Build history of the part. All positions in model axes, mm. Face numbers are marked on the shaded views. A direction names the side the tool comes from. Round coordinates to 2 decimals unless told otherwise and drop trailing zeros. Loops run counter-clockwise (first coordinate to the right, second up) from the corner with the lowest first, then second, coordinate; pieces in that order, holes last. Notation, with made-up numbers: (-4, -33.5) -> (43, -33.5) arc R30 ccw to (43, -1.5) -> close; hole circle Ø8 at (-27.75, 82). An arc over 180 degrees is marked (long way). Put each result on its own line as item: value. Start each with the question number.
Item 1: Cut at C-C, the plane y = 11.59. List the corners of the cut face in (x, z) (3 decimals).
Item 2: Tool access for the marked faces 1, 2 and 3: list every direction of +Z, -Z, +X, -X, +Y, -Y with a clear straight run to the whole face (end or side of a thin tool).
Item 3: Pull direction Y, two halves, no side cores. Call the marked faces 4, 5 and 6: +Y half, -Y half, draft (parallel to the pull), parting line (faces both ways), or undercut.
Item 4: Cut at B-B, the plane x = 3. List the corners of the cut face in (y, z), plus the area to 3 significant figures.
Item 5: Cut at D-D, the plane x = 20. List the corners of the cut face in (y, z).
Item 6: Drill centre lines: probe 1 along Y at (x, z) = (-26, 2); probe 2 along Y at (x, z) = (-4, 6.5); probe 3 along X at (y, z) = (2, 9.25). Where is each one in solid material? Low to high. Write a range as [from, to].
Item 7: Flat gauge pins, fed straight in: pin 1 Ø3 at (x, z) = (21.5, 3.5) entering from -Y; pin 2 Ø2.5 at (x, z) = (23, 8) entering from -Y; pin 3 Ø4 at (x, z) = (-24, 4.5) entering from +Y. Where does each tip first touch, or does it go through?
Item 8: Cut at A-A, the plane y = 38.79. List the corners of the cut face in (x, z) (3 decimals).
```python
from build123d import *

# Parameters (mm, degrees)
SKETCH007_W                               = 14.824166
SKETCH007_H                               = 2.145144
EXTRUDE007_DEPTH                          = 7
SKETCH006_W                               = 3.554402
SKETCH006_H                               = 1.424327
EXTRUDE006_DEPTH                          = 10
SKETCH004_AS_DRAWN_W                      = 3.541569
SKETCH004_AS_DRAWN_H                      = 1.411495
EXTRUDE005_DEPTH                          = 7
EXTRUDE005_ONTO_SKETCH004_ROLL_ANGLE      = 90
EXTRUDE005_ONTO_SKETCH004_PLACEMENT_ANGLE = 147.47511
SKETCH005_W                               = 3.573389
SKETCH005_H                               = 1.465404
EXTRUDE004_DEPTH                          = 10
SKETCH003_AS_DRAWN_W                      = 3.579881
SKETCH003_AS_DRAWN_H                      = 1.40319
EXTRUDE003_DEPTH                          = 7
EXTRUDE003_ONTO_SKETCH003_ROLL_ANGLE      = 90
EXTRUDE003_ONTO_SKETCH003_PLACEMENT_ANGLE = -147.47511
EXTRUDE002_DEPTH                          = 5
SKETCH_R                                  = 1.75
EXTRUDE_DEPTH                             = 12


with BuildPart() as extrude007:
    # Sketch007 (on Face32 of Cut004) → Extrude007 (new body)
    with BuildSketch(Plane(origin=(24, 0, 0), x_dir=(0, -1, 0), z_dir=(-1, 0, 0))):
        with Locations((-23.062542, 8.033458)):
            Rectangle(SKETCH007_W, SKETCH007_H)
    extrude(amount=-EXTRUDE007_DEPTH)


with BuildPart() as extrude006:
    # Sketch006 (on Face23 of Cut002) → Extrude006 (new body)
    with BuildSketch(Plane.XZ.offset(-36.8)):
        with Locations((-19.910848, 8.431245)):
            Rectangle(SKETCH006_W, SKETCH006_H)
    extrude(amount=-EXTRUDE006_DEPTH)


with BuildPart() as extrude005:
    # Sketch004 as drawn → Extrude005 (new)
    with BuildSketch(Plane.XY):
        with Locations((9.550918, 8.438737)):
            Rectangle(SKETCH004_AS_DRAWN_W, SKETCH004_AS_DRAWN_H)
    extrude(amount=-EXTRUDE005_DEPTH)


with BuildPart() as extrude005_1:
    # Extrude005 onto Sketch004 roll: moved
    add(extrude005.part.rotate(Axis((0, 0, 0), (1, 0, 0)), EXTRUDE005_ONTO_SKETCH004_ROLL_ANGLE))


with BuildPart() as extrude005_2:
    # Extrude005 onto Sketch004 placement: moved
    add(extrude005_1.part.moved(Location((-2.303479, -3.612274, 0))).rotate(Axis((-2.303479, -3.612274, 0), (0, 0, 1)), EXTRUDE005_ONTO_SKETCH004_PLACEMENT_ANGLE))


with BuildPart() as extrude004:
    # Sketch005 (on Face23 of Cut001) → Extrude004 (new body)
    with BuildSketch(Plane.XZ.offset(-36.8)):
        with Locations((19.895352, 8.368902)):
            Rectangle(SKETCH005_W, SKETCH005_H)
    extrude(amount=-EXTRUDE004_DEPTH)


with BuildPart() as extrude003:
    # Sketch003 as drawn → Extrude003 (new)
    with BuildSketch(Plane.XY):
        with Locations((-9.548731, 8.412013)):
            Rectangle(SKETCH003_AS_DRAWN_W, SKETCH003_AS_DRAWN_H)
    extrude(amount=-EXTRUDE003_DEPTH)


with BuildPart() as extrude003_1:
    # Extrude003 onto Sketch003 roll: moved
    add(extrude003.part.rotate(Axis((0, 0, 0), (1, 0, 0)), EXTRUDE003_ONTO_SKETCH003_ROLL_ANGLE))


with BuildPart() as extrude003_2:
    # Extrude003 onto Sketch003 placement: moved
    add(extrude003_1.part.moved(Location((2.303479, -3.612274, 0))).rotate(Axis((2.303479, -3.612274, 0), (0, 0, 1)), EXTRUDE003_ONTO_SKETCH003_PLACEMENT_ANGLE))


with BuildPart() as extrude002:
    # Sketch002 (on Face4 of Extrude) → Extrude002 (new body)
    with BuildSketch(Plane.YZ.offset(29)):
        with BuildLine():
            ThreePointArc((13.665, 7.65), (11.59, 9.725), (9.515, 7.65))
            Line((9.515, 7.65), (9.515, 2.15))
            ThreePointArc((9.515, 2.15), (11.59, 0.075), (13.665, 2.15))
            Line((13.665, 2.15), (13.665, 7.65))
        make_face()
    extrude(amount=-EXTRUDE002_DEPTH)


with BuildPart() as cut005:
    # Sketch → Extrude (new body)
    with BuildSketch(Plane.XY):
        Polygon((-21, 46.4), (21, 46.4), (21, 41.8), (29, 41.8), (29, -0.2), (21, -0.2), (6.4, -6), (-6.4, -6), (-21, -0.2), (-29, -0.2), (-29, 41.8), (-21, 41.8), align=None)
        with Locations((-25.875, 38.79)):
            Circle(SKETCH_R, mode=Mode.SUBTRACT)
        with Locations((25.875, 38.79)):
            Circle(SKETCH_R, mode=Mode.SUBTRACT)
        with Locations((25.875, 2.81)):
            Circle(SKETCH_R, mode=Mode.SUBTRACT)
        with Locations((-25.875, 2.81)):
            Circle(SKETCH_R, mode=Mode.SUBTRACT)
        with BuildLine():
            Line((-16, 41.4), (16, 41.4))
            Line((16, 41.4), (16, 36.8))
            Line((16, 36.8), (24, 36.8))
            Line((24, 36.8), (24, 4.8))
            Line((24, 4.8), (16, 4.8))
            ThreePointArc((16, 4.8), (14.479309, 4.429189), (13.3, 3.4))
            Line((6.4, -1), (13.3, 3.4))
            Line((-6.4, -1), (6.4, -1))
            Line((-6.4, -1), (-13.3, 3.4))
            ThreePointArc((-13.3, 3.4), (-14.479309, 4.429189), (-16, 4.8))
            Line((-24, 4.8), (-16, 4.8))
            Line((-24, 36.8), (-24, 4.8))
            Line((-16, 36.8), (-24, 36.8))
            Line((-16, 41.4), (-16, 36.8))
        make_face(mode=Mode.SUBTRACT)
    extrude(amount=EXTRUDE_DEPTH)

    # Cut: cut Extrude002
    add(extrude002.part, mode=Mode.SUBTRACT)

    # Cut001: cut Extrude003
    add(extrude003_2.part, mode=Mode.SUBTRACT)

    # Cut002: cut Extrude004
    add(extrude004.part, mode=Mode.SUBTRACT)

    # Cut003: cut Extrude005
    add(extrude005_2.part, mode=Mode.SUBTRACT)

    # Cut004: cut Extrude006
    add(extrude006.part, mode=Mode.SUBTRACT)

    # Cut005: cut Extrude007
    add(extrude007.part, mode=Mode.SUBTRACT)


solid = cut005.part
```
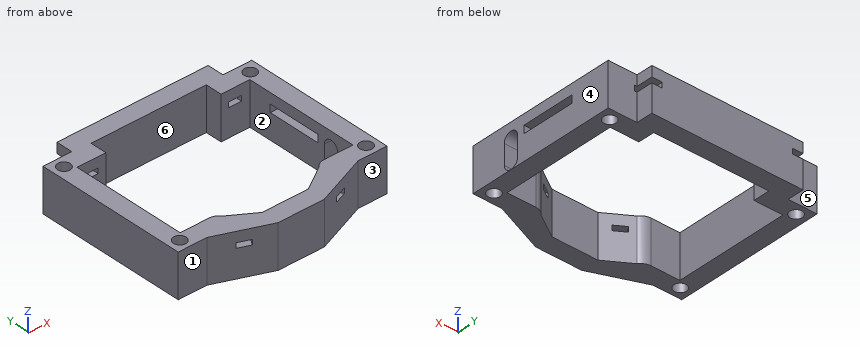
Reply:
1. outline: (-29, 0) -> (-24, 0) -> (-24, 12) -> (-29, 12) -> close; (24, 0) -> (29, 0) -> (29, 0.075) -> (24, 0.075) -> close; (24, 9.725) -> (29, 9.725) -> (29, 12) -> (24, 12) -> close
2. face 1: +Z, -Z, -X, -Y
2. face 2: +Z, -Z
2. face 3: +Z, -Z, +X, -Y
3. face 4: draft
3. face 5: +Y half
3. face 6: undercut
4. outline: (-6, 0) -> (-1, 0) -> (-1, 12) -> (-6, 12) -> close; (41.4, 0) -> (46.4, 0) -> (46.4, 12) -> (41.4, 12) -> close
4. area: 120 mm^2
5. outline: (-0.6, 0) -> (4.8, 0) -> (4.8, 12) -> (-0.6, 12) -> close; (36.8, 0) -> (46.4, 0) -> (46.4, 7.64) -> (36.8, 7.64) -> close; (36.8, 9.1) -> (46.4, 9.1) -> (46.4, 12) -> (36.8, 12) -> close
6. probe 1: y = [-0.2, 1.06], [4.56, 37.04], [40.54, 41.8]
6. probe 2: y = [-6, -1], [41.4, 46.4]
6. probe 3: x = [-29, -27.43], [-24.32, -11.1], [11.1, 24.32], [27.43, 29]
7. pin 1: stops at y = -0.6
7. pin 2: stops at y = -0.2
7. pin 3: stops at y = 41.8
8. outline: (-29, 0) -> (-27.625, 0) -> (-27.625, 12) -> (-29, 12) -> close; (-24.125, 0) -> (-16, 0) -> (-16, 12) -> (-24.125, 12) -> close; (16, 0) -> (24.125, 0) -> (24.125, 12) -> (16, 12) -> close; (27.625, 0) -> (29, 0) -> (29, 12) -> (27.625, 12) -> close; hole (-21.688, 7.719) -> (-18.134, 7.719) -> (-18.134, 9.143) -> (-21.688, 9.143) -> close; hole (18.109, 7.636) -> (21.682, 7.636) -> (21.682, 9.102) -> (18.109, 9.102) -> close
